```python
from build123d import *

# Parameters (mm, degrees)
SKETCH1_R           = 20
BOSS_EXTRUDE1_DEPTH = 165
BOSS_EXTRUDE2_START = 40
SKETCH2_R           = 15
BOSS_EXTRUDE2_DEPTH = 60
SKETCH3_W           = 206.239754747
SKETCH3_H           = 30
CUT_EXTRUDE1_DEPTH  = 173.5
SKETCH4_W           = 210
SKETCH4_H           = 170.517407572
CUT_EXTRUDE2_DEPTH  = 1054.5
FILLET1_R           = 4
FILLET2_R           = 8


with BuildPart() as part:
    # Sketch1 → Boss-Extrude1 (new, symmetric)
    with BuildSketch(Plane.XY):
        with BuildLine():
            Line((-226.495033058, 240), (-175.499287748, 240))
            ThreePointArc((-175.499287748, 240), (0, 100), (175.499287748, 240))
            Line((175.499287748, 240), (226.495033058, 240))
            ThreePointArc((226.495033058, 240), (203.453529219, 172.730892386), (160.966468811, 115.714285714))
            Line((160.966468811, 115.714285714), (20.995626367, -21.428571429))
            ThreePointArc((20.995626367, -21.428571429), (0, -30), (-20.995626367, -21.428571429))
            Line((-20.995626367, -21.428571429), (-160.966468811, 115.714285714))
            ThreePointArc((-160.966468811, 115.714285714), (-203.453529219, 172.730892386), (-226.495033058, 240))
        make_face()
        Circle(SKETCH1_R, mode=Mode.SUBTRACT)
    extrude(amount=BOSS_EXTRUDE1_DEPTH, both=True)

    # Sketch2 → Boss-Extrude2 (add)
    with BuildSketch(Plane(origin=(0, 0, 0), x_dir=(1, 0, 0), z_dir=(0, 1, 0)).offset(BOSS_EXTRUDE2_START)):
        with BuildLine():
            Line((-55, -165), (55, -165))
            Line((55, -165), (55, -205))
            Line((55, -205), (31.705882353, -254.823529412))
            ThreePointArc((31.705882353, -254.823529412), (0, -275), (-31.705882353, -254.823529412))
            Line((-31.705882353, -254.823529412), (-55, -205))
            Line((-55, -205), (-55, -165))
        make_face()
        with Locations(Location((0, -240, 0), (0, 0, 90))):
            Circle(SKETCH2_R, mode=Mode.SUBTRACT)
    extrude(amount=BOSS_EXTRUDE2_DEPTH)

    # Sketch3 → Cut-Extrude1 (cut, symmetric)
    with BuildSketch(Plane(origin=(0, 0, 0), x_dir=(0, 0, -1), z_dir=(1, 0, 0))):
        with Locations((-268.119877374, 70)):
            Rectangle(SKETCH3_W, SKETCH3_H)
    extrude(amount=CUT_EXTRUDE1_DEPTH, both=True, mode=Mode.SUBTRACT)

    # Sketch4 → Cut-Extrude2 (cut, symmetric)
    with BuildSketch(Plane(origin=(0, 0, 0), x_dir=(0, 0, -1), z_dir=(1, 0, 0))):
        with Locations((0, 9.741296214)):
            Rectangle(SKETCH4_W, SKETCH4_H)
    extrude(amount=CUT_EXTRUDE2_DEPTH, both=True, mode=Mode.SUBTRACT)

    # Fillet1
    fillet1_edges = [part.edges().sort_by_distance(p)[0] for p in [
        (0, 95, 105),
        (0, 95, -105),
    ]]
    fillet(fillet1_edges, radius=FILLET1_R)

    # Fillet2
    fillet2_edges = [part.edges().sort_by_distance(p)[0] for p in [
        (-90.981047589, 47.142857143, -165),
        (-203.453529219, 172.730892386, -165),
        (-203.453529219, 172.730892386, 165),
        (-90.981047589, 47.142857143, 165),
        (0, -30, 165),
        (90.981047589, 47.142857143, 165),
        (203.453529219, 172.730892386, 165),
        (203.453529219, 172.730892386, -165),
        (90.981047589, 47.142857143, -165),
        (0, -30, -165),
    ]]
    fillet(fillet2_edges, radius=FILLET2_R)


solid = part.part
```
The model under review builds one solid part; all positions refer to its coordinate system, in mm. A direction names the side the tool comes from. Coordinates: 2 decimals unless noted, no trailing zeros. Order: outer loops, then holes, each group sorted by start corner. A loop starts at its lowest first (then second) coordinate and runs counter-clockwise, first axis right, second up. Notation, with made-up numbers: (-3, 61) -> (26, 61) arc R18 cw to (26, 69) -> close; hole circle Ø3 at (3.5, 56.25). An arc over 180 degrees is marked (long way). Answer in a Markdown table with one row per item. Add a question column.
Item 1: Machinability: for faces 4 (the flat face through (55, 92, 185)), 5 (the flat face through (2, 57, 105)), 6 (the flat face through (1, 85, 209)), 7 (the flat face through (154.17, 109.055, 37.087)), 8 (the flat face through (1, 40, 207)), which of the approach directions +Z, -Z, +X, -X, +Y, -Y give a long, thin tool a straight path to every point of the face, cutting with its end or side? Answer none if there is none.
Item 2: We need section B-B on y = 0. Give the number of separate pieces and of enclosed holes in the cut face, plus the area to 3 significant figures.
Item 3: Mouldability with a two-part tool opening along Z and no side actions: class faces 1 (the flat face through (2, 57, -105)), 2 (the cylindrical face through (0.555, 92.395, 274.996)), 3 (the flat face through (-55, 92, 185)) as +Z half, -Z half, draft (parallel to the pull), parting line (faces both ways), or undercut.
Item 4: To check wall thickness, follow probe 1 along Y at (x, z) = (0, 139); probe 2 along X at (y, z) = (207, 74); probe 3 along X at (y, z) = (119, 54.5). State the ranges of each line that lie inside material, in increasing order.
Item 5: We need section A-A on z = 240. Write out the cut boundary in (x, y).
Item 6: Clearance check with flat-ended pins moving along their axes: pin 1 (10 mm diameter, centred on x = -37, z = 110.5, fed in from -Y); pin 2 (16.5 mm diameter, centred on y = 45, z = 191.5, fed in from +X); pin 3 (4.5 mm diameter, centred on y = 93, z = 194, fed in from -X); pin 4 (24 mm diameter, centred on x = 0, y = 0, fed in from +Z). State where each tip first meets the part, or that it passes through.
Final values:
| question | item | result |
|---|---|---|
| 1 | face 4 | +Z, +X, +Y, -Y |
| 1 | face 5 | +X, -X, -Y |
| 1 | face 6 | +Z, +X, -X |
| 1 | face 7 | +Z, -Z, +X, -Y |
| 1 | face 8 | +Z, +X, -X, -Y |
| 2 | separate pieces | 4 |
| 2 | enclosed holes | 0 |
| 2 | area | 5,410 mm2 |
| 3 | face 1 | undercut |
| 3 | face 2 | +Z half |
| 3 | face 3 | draft |
| 4 | probe 1 | y = -30 to -20, 20 to 100 |
| 4 | probe 2 | x = -218.11 to -164.53, 164.53 to 218.11 |
| 4 | probe 3 | x = -164.25 to -80.49, 80.49 to 164.25 |
| 5 | outline | (-38.64, 40) -> (-15, 40) -> (-15, 55) -> (-38.64, 55) -> close; (-38.64, 85) -> (-15, 85) -> (-15, 100) -> (-38.64, 100) -> close; (15, 40) -> (38.64, 40) -> (38.64, 55) -> (15, 55) -> close; (15, 85) -> (38.64, 85) -> (38.64, 100) -> (15, 100) -> close |
| 6 | pin 1 | stops at y = -10.65 |
| 6 | pin 2 | stops at x = 55 |
| 6 | pin 3 | stops at x = -55 |
| 6 | pin 4 | passes through |
